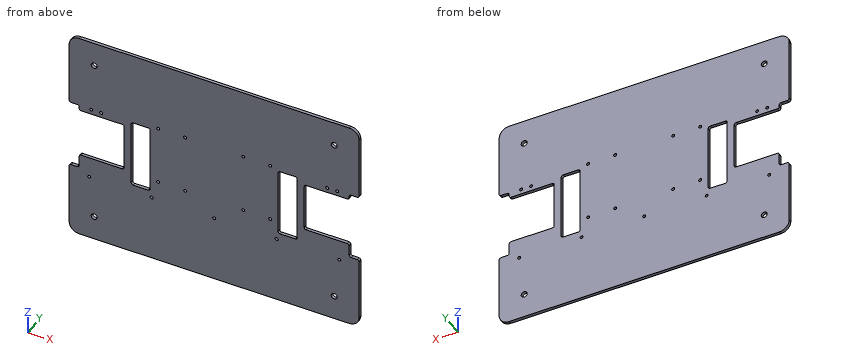
from build123d import *

# Parameters (mm, degrees)
SKETCH_1_W          = 290
SKETCH_1_H          = 220
EXTRUDE_1_DEPTH     = 3
SKETCH_2_R          = 1.5
SKETCH_2_R_2        = 3
SKETCH_2_W          = 19
SKETCH_2_H          = 70
CUT_EXTRUDE_1_DEPTH = 183.027470454
FILLET_1_R          = 10
FILLET_2_R          = 2


with BuildPart() as part:
    # Эскиз1 → Бобышка-Вытянуть1 (new body)
    with BuildSketch(Plane(origin=(0, 0, 0), x_dir=(1, 0, 0), z_dir=(0, 1, 0))):
        Rectangle(SKETCH_1_W, SKETCH_1_H)
    extrude(amount=EXTRUDE_1_DEPTH)

    # Эскиз2 → Вырез-Вытянуть1 (cut, through all)
    with BuildSketch(Plane(origin=(0, 3, 0), x_dir=(1, 0, 0), z_dir=(0, 1, 0))):
        with Locations(Location((-123, -34.3, 0), (0, 0, 270))):
            Circle(SKETCH_2_R)
        with Locations(Location((-113, -34.3, 0), (0, 0, 90))):
            Circle(SKETCH_2_R)
        with Locations(Location((123, -34.3, 0), (0, 0, 90))):
            Circle(SKETCH_2_R)
        with Locations(Location((113, -34.3, 0), (0, 0, 270))):
            Circle(SKETCH_2_R)
        with Locations(Location((-56, -38, 0), (0, 0, 270))):
            Circle(SKETCH_2_R)
        with Locations(Location((-29, -38, 0), (0, 0, 270))):
            Circle(SKETCH_2_R)
        with Locations(Location((-56, 22, 0), (0, 0, 270))):
            Circle(SKETCH_2_R)
        with Locations(Location((-29, 22, 0), (0, 0, 270))):
            Circle(SKETCH_2_R)
        with Locations(Location((56, -38, 0), (0, 0, 90))):
            Circle(SKETCH_2_R)
        with Locations(Location((29, -38, 0), (0, 0, 90))):
            Circle(SKETCH_2_R)
        with Locations(Location((29, 22, 0), (0, 0, 90))):
            Circle(SKETCH_2_R)
        with Locations(Location((56, 22, 0), (0, 0, 90))):
            Circle(SKETCH_2_R)
        with Locations(Location((-125, 42, 0), (0, 0, 270))):
            Circle(SKETCH_2_R)
        with Locations(Location((-62.5, 42, 0), (0, 0, 270))):
            Circle(SKETCH_2_R)
        with Locations(Location((0, 42, 0), (0, 0, 270))):
            Circle(SKETCH_2_R)
        with Locations(Location((125, 42, 0), (0, 0, 90))):
            Circle(SKETCH_2_R)
        with Locations(Location((62.5, 42, 0), (0, 0, 90))):
            Circle(SKETCH_2_R)
        with Locations(Location((-120, 85, 0), (0, 0, 270))):
            Circle(SKETCH_2_R_2)
        with Locations(Location((-120, -85, 0), (0, 0, 270))):
            Circle(SKETCH_2_R_2)
        with Locations(Location((120, 85, 0), (0, 0, 90))):
            Circle(SKETCH_2_R_2)
        with Locations(Location((120, -85, 0), (0, 0, 90))):
            Circle(SKETCH_2_R_2)
        Polygon((135, -35), (145, -35), (145, 35), (135, 35), (135, 20.7), (90, 20.7), (90, -29.3), (135, -29.3), align=None)
        Polygon((-135, -35), (-145, -35), (-145, 35), (-135, 35), (-135, 20.7), (-90, 20.7), (-90, -29.3), (-135, -29.3), align=None)
        with Locations((73.5, 0)):
            Rectangle(SKETCH_2_W, SKETCH_2_H)
        with Locations((-73.5, 0)):
            Rectangle(SKETCH_2_W, SKETCH_2_H)
    extrude(amount=-CUT_EXTRUDE_1_DEPTH, mode=Mode.SUBTRACT)

    # Скругление1
    fillet_1_edges = [part.edges().sort_by_distance(p)[0] for p in [
        (145, 1.5, 110),
        (-145, 1.5, 110),
        (-145, 1.5, -110),
        (145, 1.5, -110),
    ]]
    fillet(fillet_1_edges, radius=FILLET_1_R)

    # Скругление2
    fillet_2_edges = [part.edges().sort_by_distance(p)[0] for p in [
        (-145, 1.5, 35),
        (-145, 1.5, -35),
        (-135, 1.5, -35),
        (-135, 1.5, -20.7),
        (-90, 1.5, -20.7),
        (-90, 1.5, 29.3),
        (-135, 1.5, 29.3),
        (-135, 1.5, 35),
        (135, 1.5, 35),
        (135, 1.5, 29.3),
        (90, 1.5, 29.3),
        (90, 1.5, -20.7),
        (135, 1.5, -20.7),
        (135, 1.5, -35),
        (145, 1.5, -35),
        (145, 1.5, 35),
        (-64, 1.5, -35),
        (-64, 1.5, 35),
        (-83, 1.5, 35),
        (-83, 1.5, -35),
        (83, 1.5, -35),
        (83, 1.5, 35),
        (64, 1.5, 35),
        (64, 1.5, -35),
    ]]
    fillet(fillet_2_edges, radius=FILLET_2_R)


solid = part.part
Here's how the part is built. I have some questions about the finished solid (model axes, mm). Round coordinates to 2 decimals unless told otherwise and drop trailing zeros. Write each loop counter-clockwise with the first axis right and the second up, starting at its lowest first coordinate (ties: lowest second). Pieces come first, ordered by that corner, then holes. Notation, with made-up numbers: (14, 22.25) -> (73, 22.25) arc R9 ccw to (73, 28.25) -> close; hole circle Ø9 at (17.5, -4.75). An arc over 180 degrees is marked (long way). One line per item, written item: value.
1) I'm going to push flat-ended pins straight in: pin 1 Ø1.5 at (x, y) = (141, 1) entering from +Z; pin 2 Ø1.5 at (y, z) = (1, -29) entering from +X; pin 3 Ø1 at (y, z) = (1, 6.5) entering from -X. Where does each tip first touch, or does it pass through?
Filled sheet:
pin 1: stops at z = 108.51
pin 2: stops at x = 135
pin 3: stops at x = -90
2) Suppose I cut it at B-B on z = -85. List the corners of the cut face in (x, y) for me, plus the area to 3 significant figures.
Filled sheet:
outline: (-145, 0) -> (-123, 0) -> (-123, 3) -> (-145, 3) -> close; (-117, 0) -> (117, 0) -> (117, 3) -> (-117, 3) -> close; (123, 0) -> (145, 0) -> (145, 3) -> (123, 3) -> close
area: 834 mm2
3) Suppose I cut it at A-A on z = 2. List the corners of the cut face in (x, y) for me, plus the area to 3 significant figures.
Filled sheet:
outline: (-90, 0) -> (-83, 0) -> (-83, 3) -> (-90, 3) -> close; (-64, 0) -> (64, 0) -> (64, 3) -> (-64, 3) -> close; (83, 0) -> (90, 0) -> (90, 3) -> (83, 3) -> close
area: 426 mm2
4) Suppose I cut it at C-C on y = 0.75. Give the number of separate pieces and of enclosed holes in the cut face, plus the area to 3 significant figures.
Filled sheet:
separate pieces: 1
enclosed holes: 23
area: 54,900 mm2
5) If I drill on line 1 (Z direction, x = 29, y = 2.45); line 2 (X direction, y = 1.2, z = 16.5); line 3 (Z direction, x = -113, y = 1.4), over which ranges is the centre line in solid material (lowest first)? Write a range as [from, to].
Filled sheet:
line 1: z = [-110, -23.5], [-20.5, 36.5], [39.5, 110]
line 2: x = [-90, -83], [-64, 64], [83, 90]
line 3: z = [-110, -20.7], [29.3, 32.8], [35.8, 110]
